Autodesk Inventor part; units mm, degrees
ref_plane "YZ Plane" through (0, 0, 0) normal (1, 0, 0) x (0, 1, 0)
ref_plane "XZ Plane" through (0, 0, 0) normal (0, 1, 0) x (-1, 0, 0)
ref_plane "XY Plane" through (0, 0, 0) normal (0, 0, 1) x (1, 0, 0)
sketch "Sketch1" plane through (0, 0, 0) normal (0, 1, 0) x (-1, 0, 0)
  line L0 (30, -10) -> (-30, -10)
  line L1 (-40, 0) -> (-40, 0)
  line L2 (-30, 10) -> (30, 10)
  line L3 (40, 0) -> (40, 0)
  line L4 (40, -10) -> (-40, 10) construction
  line L5 (-40, -10) -> (40, 10) construction
  line L6 (0, 0) -> (35, 0)
  line L7 (0, 0) -> (35, 0) construction
  line L8 (0, 0) -> (-35, 0) construction
  line L9 (0, 0) -> (35, 0) construction
  circle A0 centre (35, 0) radius 1.5
  circle A1 centre (-35, 0) radius 1.5
  arc A2 (-30, 10) -> (-40, 0) centre (-30, 0) ccw
  arc A3 (-40, 0) -> (-30, -10) centre (-30, 0) ccw
  arc A4 (30, -10) -> (40, 0) centre (30, 0) ccw
  arc A5 (40, 0) -> (30, 10) centre (30, 0) ccw
  point P0 (40, 0)
  point P1 (-40, 0)
  dimension "d0" = 80
  dimension "d1" = 20
  dimension "d3" = 35
  dimension "d4" = 0
  dimension "d5" = 35
  dimension "d6" = 180
  dimension "d7" = 3
  dimension "d8" = 3
  dimension "d11" = 10
extrude "Extrusion1" add sketch "Sketch1" along normal blind 6
properties part number "fuselagewingconnection"
For this review, take the finished solid that the model builds, in its own axes (mm). Give positions to 0.01 mm unless a question says otherwise; leave off trailing zeros. Loops run counter-clockwise (first coordinate to the right, second up) from the corner with the lowest first, then second, coordinate; pieces in that order, holes last. Notation, with made-up numbers: M 72.5,-11.5 L 98.5,-11.5 A13 ccw 98.5,10.5 Z; hole C 41,48.5 d3. An arc over 180 degrees is marked long. One line per item, written item: value. Start each with the question number.
Q1. Add section D-D (z = 4.75). Give the boundary of the cut face in (x, y).
Q2. Add section C-C (x = 35). Give the boundary of the cut face in (y, z), and give its area (3 significant figures).
Q3. Add section B-B (z = 0.75). Give the boundary of the cut face in (x, y), and give its area (3 significant figures).
Q4. Draft analysis for pull direction X (two halves, no side actions). For faces 1 (the face through (-40, 3, 0)), 2 (the face through (1, 0, 0)), 3 (the face through (-33.8, 3, 0.9)), state which applies: released by +X, released by -X, zero draft, split by the parting line, or undercut.
Q5. Add section A-A (y = 1.2). Give the boundary of the cut face in (x, z).
Q6. For L1, parallel to X at y = 4.2, z = -1.25; L2, parallel to Z at x = -35, y = 1.95; L3, parallel to X at y = 0.4, z = 0.75, list the stretches that pass through material, from the lowest coordinate up.
Reply:
1. outline: M -38.8,0 L 38.8,0 L 38.8,6 L -38.8,6 Z
2. outline: M 0,-8.66 L 6,-8.66 L 6,-1.5 L 0,-1.5 Z; M 0,1.5 L 6,1.5 L 6,8.66 L 0,8.66 Z
2. area: 85.9 mm²
3. outline: M -39.97,0 L -36.3,0 L -36.3,6 L -39.97,6 Z; M -33.7,0 L 33.7,0 L 33.7,6 L -33.7,6 Z; M 36.3,0 L 39.97,0 L 39.97,6 L 36.3,6 Z
3. area: 448 mm²
4. face 1: released by -X
4. face 2: zero draft
4. face 3: undercut
5. outline: M -30,-10 L 30,-10 A10 ccw 30,10 L -30,10 A10 ccw Z; hole C -35,0 d3; hole C 35,0 d3
6. L1: -39.92 to -35.83, -34.17 to 34.17, 35.83 to 39.92
6. L2: -8.66 to -1.5, 1.5 to 8.66
6. L3: -39.97 to -36.3, -33.7 to 33.7, 36.3 to 39.97
